Verification items for the finished model (mm, model axes). A direction names the side the tool comes from. Round coordinates to 2 decimals unless told otherwise and drop trailing zeros. Write each loop counter-clockwise with the first axis right and the second up, starting at its lowest first coordinate (ties: lowest second). Pieces come first, ordered by that corner, then holes. Notation, with made-up numbers: (62, -25) -> (87, -25) arc R18 ccw to (87, -16) -> close; hole circle Ø2 at (11, 20). An arc over 180 degrees is marked (long way). Answer as a JSON object with one key per item and string values. Group by question number.
(1) Scan lines: L1, parallel to Y at x = 450.38, z = 0.8; L2, parallel to X at y = 75.5, z = 1.05; L3, parallel to X at y = 71, z = 1.7. Record each from-to range of solid material in increasing order. Write a range as from..to.
(2) Gauge pin test, flat ends, axial feed: pin 1 Ø10 at (x, y) = (193.5, 21) entering from -Z; pin 2 Ø1 at (x, z) = (273.5, 1.5) entering from +Y; pin 3 Ø1 at (y, z) = (73.5, 1) entering from +X; pin 4 Ø1 at (x, z) = (153.5, 0.5) entering from +Y. Record the tip position at first contact, or that the pin passes through.
(3) Set-up check for faces 1 (the face through (261.287, 83.39, 1.014)), 2 (the face through (291.13, 61.25, 1.01)): record each of +Z, -Z, +X, -X, +Y, -Y from which the full face is reachable in a straight line by a thin tool's end or side.
(4) Sectioned sample at B-B on x = 122.5. Record the cut outline in (y, z), and give its area (3 significant figures).
(5) Sectioned sample at A-A on z = 1.1. Count the separate pieces of the cut face and the enclosed holes in it, and give its area (3 significant figures).
Autodesk Inventor part; units mm, degrees
ref_plane "YZ Plane" through (0, 0, 0) normal (1, 0, 0) x (0, 1, 0)
ref_plane "XZ Plane" through (0, 0, 0) normal (0, 1, 0) x (-1, 0, 0)
ref_plane "XY Plane" through (0, 0, 0) normal (0, 0, 1) x (1, 0, 0)
sketch "Szkic1" plane through (0, 0, 0) normal (0, 0, 1) x (1, 0, 0)
  line L0 (-98.62, 58.242) -> (467.38, 58.242)
  line L1 (467.38, 58.242) -> (467.38, -3.758)
  line L2 (467.38, -3.758) -> (-98.62, -3.758)
  line L3 (-98.62, -3.758) -> (-98.62, 58.242)
  line L4 (65.48, 58.242) -> (95.48, 58.242)
  line L5 (95.48, 58.242) -> (95.48, 86.242)
  line L6 (95.48, 86.242) -> (65.48, 86.242)
  line L7 (65.48, 86.242) -> (65.48, 58.242)
  line L8 (258.28, 58.242) -> (288.28, 58.242)
  line L9 (288.28, 58.242) -> (288.28, 86.242)
  line L10 (288.28, 86.242) -> (258.28, 86.242)
  line L11 (258.28, 86.242) -> (258.28, 58.242)
  line L12 (-98.62, 58.242) -> (-68.62, 58.242)
  line L13 (-68.62, 58.242) -> (-68.62, 88.242)
  line L14 (-68.62, 88.242) -> (-98.62, 88.242)
  line L15 (-98.62, 88.242) -> (-98.62, 58.242)
  point P0 (0, 0)
  point P1 (80.48, 71.242)
  point P2 (273.28, 71.242)
  point P3 (-81.62, 68.242)
  point P4 (450.38, 43.242)
  point P5 (-81.62, 11.242)
  point P6 (450.38, 11.242)
  dimension "d0" = 566
  dimension "d1" = 62
  dimension "d2" = 30
  dimension "d3" = 28
  dimension "d4" = 30
  dimension "d5" = 28
  dimension "d6" = 164.1
  dimension "d7" = 356.9
  dimension "d11" = 15
  dimension "d12" = 15
  dimension "d13" = 15
  dimension "d14" = 15
  dimension "d16" = 15
  dimension "d17" = 17
  dimension "d18" = 17
  dimension "d26" = 17
  dimension "d27" = 15
  dimension "d28" = 17
  dimension "d29" = 15
  dimension "d30" = 30
  dimension "d31" = 30
  dimension "d33" = 20
extrude "Wyciągnięcie proste1" add sketch "Szkic1" along normal blind 2
fillet "Zaokrąglenie1" radius 10 8 edges at (258.28, 58.242, 1) (258.28, 86.242, 1) (288.28, 86.242, 1) (288.28, 58.242, 1) (95.48, 58.242, 1) (95.48, 86.242, 1) (65.48, 86.242, 1) (65.48, 58.242, 1)
hole "Otwór1" at (80.48, 71.242, 0) at (273.28, 71.242, 0) at (-81.62, 68.242, 0) at (450.38, 43.242, 0) at (-81.62, 11.242, 0) at (450.38, 11.242, 0) direction (0, 0, 1) diameter 4 end through all
fillet "Zaokrąglenie2" radius 30 2 edges at (-68.62, 58.242, 1) (-68.62, 88.242, 1)
equation "\"d3\" = d5"
properties part number "LC_ALU_2mm_Right_Plate"
Computed values:
{
 "1": {"L1": "-3.76..9.24, 13.24..41.24, 45.24..58.24", "L2": "-98.62..-66.04, 65.48..95.48, 258.28..288.28", "L3": "-98.62..-63.17, 65.48..78.49, 82.47..95.48, 258.28..271.29, 275.27..288.28"},
 "2": {"pin 1": "z = 0", "pin 2": "y = 86.24", "pin 3": "x = 288.28", "pin 4": "y = 58.24"},
 "3": {"face 1": "+Z, -Z, +Y", "face 2": "+Z, -Z, +X, +Y"},
 "4": {"outline": "(-3.76, 0) -> (58.24, 0) -> (58.24, 2) -> (-3.76, 2) -> close", "area": "124 mm2"},
 "5": {"separate pieces": "1", "enclosed holes": "6", "area": "37,700 mm2"}
}
